Part model, mm, in its own coordinate system. Face numbers are marked on the shaded views. A direction names the side the tool comes from. Round coordinates to 2 decimals unless told otherwise and drop trailing zeros. Write each loop counter-clockwise with the first axis right and the second up, starting at its lowest first coordinate (ties: lowest second). Pieces come first, ordered by that corner, then holes. Notation, with made-up numbers: (-18, -6) -> (18, -6) arc R25 ccw to (18, 25) -> close; hole circle Ø9 at (39, 77.25). An arc over 180 degrees is marked (long way). Use CSV: the item, a comma, the result in double quotes. Start each with the question number.
(1) Which spindle directions (+Z, -Z, +X, -X, +Y, -Y) get a long thin tool onto all of the face, cutting with end or side? Do the marked faces 1 and 2. Say none if no direction does.
(2) Saw through at C-C (z = -43). Give the cut face in (x, y), plus the area to 3 significant figures.
(3) Saw through at A-A (x = 0). Give the cut face in (y, z).
(4) Probe line 1 (Z direction, x = 0, y = 1.5); line 2 (X direction, y = 6, z = -7); line 3 (X direction, y = 1, z = -24). List the from-to ranges inside material, lowest first. Write a range as [from, to].
(5) Saw through at D-D (x = -14). Give the cut face in (y, z).
(6) Drop flat-ended pins along their axis: pin 1 (3 mm diameter, centred on x = 0, z = -53, fed in from +Y); pin 2 (6 mm diameter, centred on y = 4, z = -18.5, fed in from +X); pin 3 (2 mm diameter, centred on y = 6.5, z = -50.5, fed in from -X); pin 4 (4 mm diameter, centred on x = 0, z = -21.2, fed in from +Y). Give the stop position or say it passes through.
(7) Saw through at B-B (y = 1.75). Count the separate pieces of the cut face and the enclosed holes in it, plus the area to 3 significant figures.
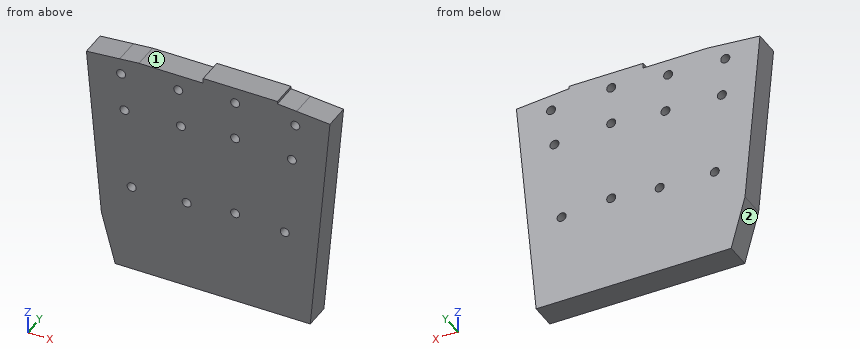
Autodesk Inventor part; units mm, degrees
ref_plane "Work Plane1" through (-22.5, 0, -2) normal (-0.0697565, 0, 0.9975641) x (0, -1, 0)
ref_plane "YZ Plane" through (0, 0, 0) normal (1, 0, 0) x (0, 1, 0)
ref_plane "XZ Plane" through (0, 0, 0) normal (0, 1, 0) x (-1, 0, 0)
sketch "Sketch1" plane through (0, 0, 0) normal (0, 1, 0) x (-1, 0, 0)
  line L0 (77, 0) -> (-56, 0)
  line L1 (0, -111.5403) -> (0, 39.2421) construction
  line L2 (58, 0) -> (-37, 0) construction
  line L3 (-37, 0) -> (-29.126, -90)
  line L4 (-29.126, -90) -> (46.5168, -90)
  line L5 (46.5168, -90) -> (51.8758, -70)
  line L6 (51.8758, -70) -> (58, 0)
  line L7 (0, -90) -> (0, -90) construction
  line L8 (-16.126, -90) -> (-24.0526, 0.6013) construction
  line L9 (37.126, -90) -> (46.4907, 17.039) construction
  circle A0 centre (44.2275, -8.8301) radius 1.75
  circle A1 centre (22.0675, -8.1849) radius 1.75
  circle A2 centre (0, -6.2) radius 1.75
  circle A3 centre (-23.315, -7.8301) radius 1.75
  circle A4 centre (42.9201, -23.773) radius 1.75
  circle A5 centre (21.0212, -23.1484) radius 1.75
  circle A6 centre (0, -21.2) radius 1.75
  circle A7 centre (-22.0076, -22.773) radius 1.75
  circle A8 centre (40.1486, -55.452) radius 1.75
  circle A9 centre (18.8029, -54.8709) radius 1.75
  circle A10 centre (0, -53) radius 1.75
  circle A11 centre (-19.2361, -54.452) radius 1.75
  line L10 (44.2275, -8.8301) -> (42.9201, -23.773)
  line L11 (22.0675, -8.1849) -> (21.0212, -23.1484)
  line L12 (0, -21.2) -> (0, -6.2)
  line L13 (-22.0076, -22.773) -> (-23.315, -7.8301)
  line L14 (42.9201, -23.773) -> (40.1486, -55.452)
  line L15 (0, -21.2) -> (0, -53)
  line L16 (-19.2361, -54.452) -> (-22.0076, -22.773)
  line L17 (21.0212, -23.1484) -> (18.8029, -54.8709)
  line L18 (12.3839, 0) -> (-16.3839, 0)
  line L19 (-16.3839, 0) -> (-16.3839, -1)
  line L20 (-16.3839, -1) -> (-36.7566, -2.7824)
  line L21 (12.3839, 0) -> (12.3839, -2)
  line L22 (12.3839, -2) -> (37.2964, -2)
  line L23 (37.2964, -2) -> (57.6691, -3.7824)
  line L24 (0, -6.2) -> (0, 0)
  line L25 (22.0675, -8.1849) -> (22.5, -2)
  line L26 (44.2275, -8.8301) -> (44.7678, -2.6537)
  line L27 (-23.315, -7.8301) -> (-23.8553, -1.6537)
  line L28 (16.3464, -90) -> (23.8777, 17.7017) construction
  point P0 (-24, 0)
  point P1 (25, 0)
  point P2 (45, 0)
  dimension "d0" = 95
  dimension "d1" = 37
  dimension "d2" = 24
  dimension "d3" = 25
  dimension "d4" = 45
  dimension "d5" = 5
  dimension "d7" = 5
  dimension "d8" = 105
  dimension "d9" = 20
  dimension "d10" = 90
  dimension "d11" = 3.5
  dimension "d12" = 31.8
  dimension "d13" = 15
  dimension "d14" = 2
  dimension "d15" = 1
  dimension "d16" = 7.5
  dimension "d18" = 7.5
  dimension "d19" = 6.2
  dimension "d22" = 4
  dimension "d23" = 22.5
extrude "Extrusion1" add sketch "Sketch1" along normal blind 10 contours L21 L22 L23 L6 L5 L4 L3 L20 L19 L0
ref_plane "Work Plane1" through (-22.5, 0, -2) normal (-0.0697565, 0, 0.9975641) x (0, -1, 0)
properties part number "empty"
Answers:
1,face 1,"+Z, -X, +Y, -Y"
1,face 2,"-Z, -X, +Y, -Y"
2,outline,"(-54.24, 0) -> (33.24, 0) -> (33.24, 10) -> (-54.24, 10) -> close"
2,area,"875 mm²"
3,outline,"(0, -90) -> (10, -90) -> (10, -54.75) -> (0, -54.75) -> close; (0, -51.25) -> (10, -51.25) -> (10, -22.95) -> (0, -22.95) -> close; (0, -19.45) -> (10, -19.45) -> (10, -7.95) -> (0, -7.95) -> close; (0, -4.45) -> (10, -4.45) -> (10, 0) -> (0, 0) -> close"
4,line 1,"z = [-90, -54.75], [-51.25, -22.95], [-19.45, -7.95], [-4.45, 0]"
4,line 2,"x = [-57.39, -23.36], [-20.78, -1.56], [1.56, 21.77], [24.86, 36.39]"
4,line 3,"x = [-55.9, -44.66], [-41.18, -22.55], [-19.49, 20.76], [23.26, 34.9]"
5,outline,"(0, -90) -> (10, -90) -> (10, -2) -> (0, -2) -> close"
6,pin 1,"passes through"
6,pin 2,"stops at x = 35.64"
6,pin 3,"stops at x = -53.67"
6,pin 4,"stops at y = 10"
7,separate pieces,"1"
7,enclosed holes,"12"
7,area,"7,540 mm²"
